Can you work these out from the drawing? Everything is in mm from the part's minimum corner. Give positions to 0.01 mm unless a question says otherwise; leave off trailing zeros. Loops run counter-clockwise (first coordinate to the right, second up) from the corner with the lowest first, then second, coordinate; pieces in that order, holes last. Notation, with made-up numbers: (-32.75, -23) - (-19.75, -23) arc R8 ccw to (-19.75, -8) - close; hole circle Ø11 at (-1, 27). An arc over 180 degrees is marked (long way). Write each question's results on one line, items separated by ' | '. Start each with the question number.
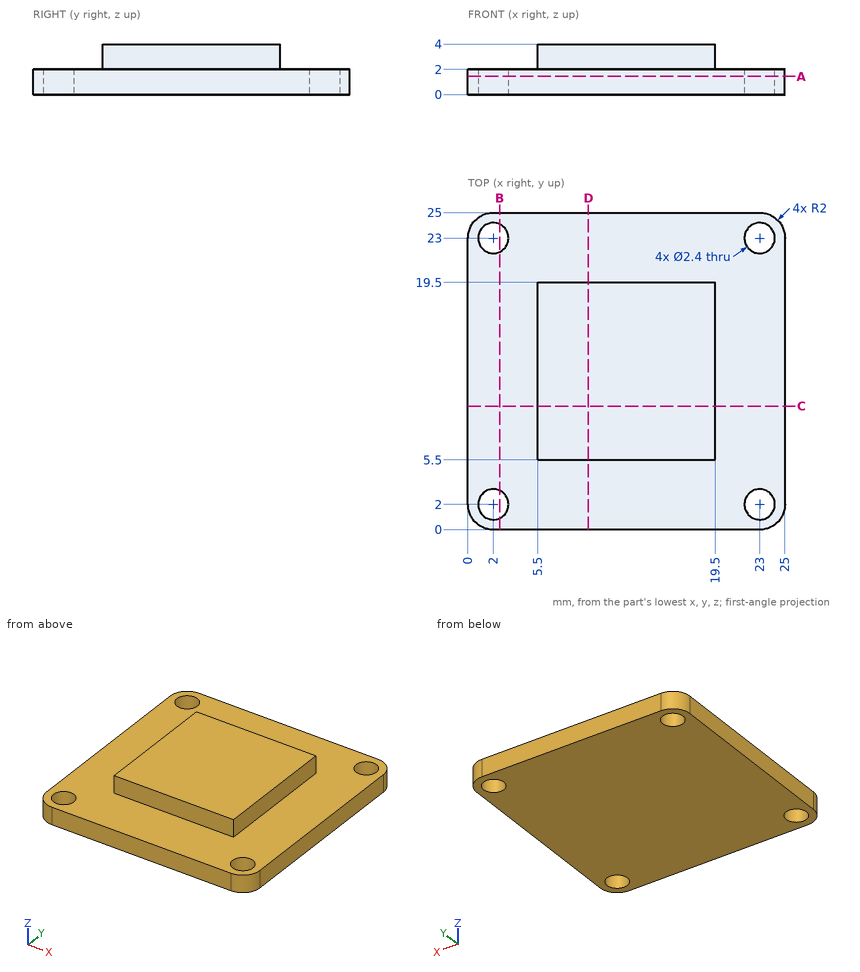
Q1. I want a section at B-B, the plane x = 2.5. List the corners of the cut face in (y, z) for me.
Q2. I'm going to push flat-ended pins straight in: pin 1 Ø2 at (x, y) = (23, 23) entering from +Z; pin 2 Ø1.6 at (x, z) = (10, 3) entering from +Y; pin 3 Ø2 at (y, z) = (16, 3.5) entering from -X; pin 4 Ø3 at (x, y) = (23, 2) entering from +Z. Where does each tip first touch, or does it pass through?
Q3. I want a section at C-C, the plane y = 9.75. List the corners of the cut face in (x, z) for me, then the cut area to 3 significant figures.
Q4. I want a section at A-A, the plane z = 1.45. List the corners of the cut face in (x, y) for me, then the cut area to 3 significant figures.
Q5. I need wall thicknesses on L1, parallel to Y at x = 2, z = 1.65; L2, parallel to X at y = 12.5, z = 2.4; L3, parallel to Z at x = 20.25, y = 12.5. Which ranges of each line are inside material? Lowest first, please. Write a range as from..to.
Conclusion:
1) outline: (0, 0) - (0.91, 0) - (0.91, 2) - (0, 2) - close; (3.09, 0) - (21.91, 0) - (21.91, 2) - (3.09, 2) - close; (24.09, 0) - (25, 0) - (25, 2) - (24.09, 2) - close
2) pin 1: through | pin 2: y = 19.5 | pin 3: x = 5.5 | pin 4: z = 2
3) outline: (0, 0) - (25, 0) - (25, 2) - (19.5, 2) - (19.5, 4) - (5.5, 4) - (5.5, 2) - (0, 2) - close | area: 78.0 mm^2
4) outline: (0, 2) arc R2 ccw to (2, 0) - (23, 0) arc R2 ccw to (25, 2) - (25, 23) arc R2 ccw to (23, 25) - (2, 25) arc R2 ccw to (0, 23) - close; hole circle Ø2.4 at (2, 2); hole circle Ø2.4 at (2, 23); hole circle Ø2.4 at (23, 2); hole circle Ø2.4 at (23, 23) | area: 603 mm^2
5) L1: 0..0.8, 3.2..21.8, 24.2..25 | L2: 5.5..19.5 | L3: 0..2
